```python
from build123d import *

# Parameters (mm, degrees)
SKETCH1_W      = 35
SKETCH1_H      = 10
EXTRUDE1_DEPTH = 38
SKETCH2_W      = 31
SKETCH2_H      = 8
EXTRUDE2_DEPTH = 30
FILLET1_R      = 2
SKETCH3_R      = 2.5
EXTRUDE3_DEPTH = 34
SKETCH4_R      = 2.5
EXTRUDE4_DEPTH = 36


with BuildPart() as part:
    # Sketch1 → Extrude1 (new body)
    with BuildSketch(Plane(origin=(0, 0, 0), x_dir=(0, 0, -1), z_dir=(1, 0, 0))):
        with Locations((-56.771768295, 48.134111791)):
            Rectangle(SKETCH1_W, SKETCH1_H)
    extrude(amount=EXTRUDE1_DEPTH)

    # Sketch2 → Extrude2 (add)
    with BuildSketch(Plane(origin=(38, 0, 0), x_dir=(0, 0, -1), z_dir=(1, 0, 0))):
        with Locations((-56.771768295, 49.134111791)):
            Rectangle(SKETCH2_W, SKETCH2_H)
    extrude(amount=EXTRUDE2_DEPTH)

    # Fillet1
    fillet1_edges = [part.edges().sort_by_distance(p)[0] for p in [
        (53, 45.134111791, 72.271768295),
        (53, 45.134111791, 41.271768295),
    ]]
    fillet(fillet1_edges, radius=FILLET1_R)

    # Sketch3 → Extrude3 (cut, through all)
    with BuildSketch(Plane(origin=(0, 0, 41.271768295), x_dir=(-1, 0, 0), z_dir=(0, 0, -1))):
        with Locations((-63, 48.134111791)):
            Circle(SKETCH3_R)
        with Locations((-53, 48.134111791)):
            Circle(SKETCH3_R)
    extrude(amount=-EXTRUDE3_DEPTH, mode=Mode.SUBTRACT)

    # Sketch4 → Extrude4 (cut, through all)
    with BuildSketch(Plane(origin=(0, 0, 39.271768295), x_dir=(-1, 0, 0), z_dir=(0, 0, -1))):
        with Locations((-4, 48.134111791)):
            Circle(SKETCH4_R)
    extrude(amount=-EXTRUDE4_DEPTH, mode=Mode.SUBTRACT)


solid = part.part
```
Geometry: final body of the model. Coordinates: model frame, mm. A direction names the side the tool comes from. Round coordinates to 2 decimals unless told otherwise and drop trailing zeros. Write each loop counter-clockwise with the first axis right and the second up, starting at its lowest first coordinate (ties: lowest second). Pieces come first, ordered by that corner, then holes.
Item 1: Material intervals for L1, parallel to X at y = 48, z = 47.5; L2, parallel to X at y = 46.25, z = 67.5; L3, parallel to Y at x = 63, z = 54.5, sorted ascending.
Item 2: Section query A-A (x = 4). Return loops of the section in (y, z).
Item 3: Section query D-D (x = 58.5). Return loops of the section in (y, z), plus the area to 3 significant figures.
Item 4: Mould query, pull axis X, two halves, no side actions, for faces 5 (the face through (0, 48, 57)), 6 (the face through (2.656, 50.242, 56.527)), 7 (the face through (53, 51, 41.272)). Classes: +X half, -X half, draft (parallel to the pull), parting line (faces both ways), or undercut.
Item 5: Section query C-C (z = 58). Return loops of the section in (x, y).
Item 6: Pin query (flat end, axial travel): P1, Ø3, axis at x = 49.5, y = 50.5, coming from the -Z side; P2, Ø6, axis at x = 57, y = 48, coming from the +Z side. Return the tip coordinate at first contact, or that it passes through.
Item 7: Set-up query: faces 1 (the face through (53.21, 45.331, 71.137)), 2 (the face through (38, 44.8, 58.1)), 3 (the face through (53.21, 45.483, 42.143)), 4 (the face through (53, 51, 72.272)). Return all of +Z, -Z, +X, -X, +Y, -Y with unobstructed straight access to the full face (end or side cutting, diameter ignored); none if empty.
Item 8: Section query B-B (y = 52.5). Return loops of the section in (x, z).
Completed:
1. L1: x = 0 to 1.5, 6.5 to 50.5, 55.5 to 60.5, 65.5 to 68
1. L2: x = 0 to 2.36, 5.64 to 51.36, 54.64 to 61.36, 64.64 to 68
1. L3: y = 45.13 to 45.63, 50.63 to 53.13
2. outline: (43.13, 39.27) - (45.63, 39.27) - (45.63, 74.27) - (43.13, 74.27) - close; (50.63, 39.27) - (53.13, 39.27) - (53.13, 74.27) - (50.63, 74.27) - close
3. outline: (45.13, 43.27) arc R2 ccw to (47.13, 41.27) - (53.13, 41.27) - (53.13, 72.27) - (47.13, 72.27) arc R2 ccw to (45.13, 70.27) - close
3. area: 246 mm2
4. face 5: -X half
4. face 6: undercut
4. face 7: draft
5. outline: (0, 43.13) - (38, 43.13) - (38, 45.13) - (68, 45.13) - (68, 53.13) - (0, 53.13) - close; hole circle Ø5 at (4, 48.13); hole circle Ø5 at (53, 48.13); hole circle Ø5 at (63, 48.13)
6. P1: stops at z = 41.27
6. P2: stops at z = 72.27
7. face 1: +Z, +X, -Y
7. face 2: +X, -Y
7. face 3: -Z, +X, -Y
7. face 4: +Z, +X, +Y, -Y
8. outline: (0, 39.27) - (38, 39.27) - (38, 41.27) - (68, 41.27) - (68, 72.27) - (38, 72.27) - (38, 74.27) - (0, 74.27) - close
